```python
from build123d import *

# Parameters (mm, degrees)
BOSS_EXTRUDE1_DEPTH = 12.7
CUT_EXTRUDE1_DEPTH  = 10.795
SKETCH3_R           = 3.175
CUT_EXTRUDE2_DEPTH  = 23.622
SKETCH4_R           = 1.905
CUT_EXTRUDE3_DEPTH  = 7.62
SKETCH5_R           = 4.445
CUT_EXTRUDE4_DEPTH  = 1.27


with BuildPart() as part:
    # Sketch1 → Boss-Extrude1 (new body)
    with BuildSketch(Plane.XY):
        with BuildLine():
            Line((-15.875, 241.3), (-15.875, 41.885940063))
            ThreePointArc((-15.875, 41.885940063), (-17.859739298, 27.82498979), (-23.658870968, 14.862752926))
            ThreePointArc((-23.658870968, 14.862752926), (0, -27.94), (23.658870968, 14.862752926))
            ThreePointArc((23.658870968, 14.862752926), (17.859739298, 27.82498979), (15.875, 41.885940063))
            Line((15.875, 41.885940063), (15.875, 241.3))
            ThreePointArc((15.875, 241.3), (0, 257.175), (-15.875, 241.3))
        make_face()
    extrude(amount=BOSS_EXTRUDE1_DEPTH)

    # Sketch2 → Cut-Extrude1 (cut)
    with BuildSketch(Plane.XY.offset(12.7)):
        with BuildLine():
            Line((-11.43, 234.95), (11.43, 234.95))
            ThreePointArc((11.43, 234.95), (13.226051224, 234.206051224), (13.97, 232.41))
            Line((13.97, 232.41), (13.97, 41.885940063))
            ThreePointArc((13.97, 41.885940063), (16.029167022, 27.297704155), (22.045766129, 13.849383408))
            ThreePointArc((22.045766129, 13.849383408), (0, -26.035), (-22.045766129, 13.849383408))
            ThreePointArc((-22.045766129, 13.849383408), (-16.029167022, 27.297704155), (-13.97, 41.885940063))
            Line((-13.97, 41.885940063), (-13.97, 232.41))
            ThreePointArc((-13.97, 232.41), (-13.226051224, 234.206051224), (-11.43, 234.95))
        make_face()
    extrude(amount=-CUT_EXTRUDE1_DEPTH, mode=Mode.SUBTRACT)

    # Sketch3 → Cut-Extrude2 (cut)
    with BuildSketch(Plane.XY.offset(12.7)):
        with Locations((0, 241.3)):
            Circle(SKETCH3_R)
    extrude(amount=-CUT_EXTRUDE2_DEPTH, mode=Mode.SUBTRACT)

    # Sketch4 → Cut-Extrude3 (cut)
    with BuildSketch(Plane.XY.offset(12.7)):
        with Locations((-11.405580841, 241.3)):
            Circle(SKETCH4_R)
        with Locations((-9.877522754, 247.002790421)):
            Circle(SKETCH4_R)
        with Locations((-5.702790421, 251.177522754)):
            Circle(SKETCH4_R)
        with Locations((0, 252.705580841)):
            Circle(SKETCH4_R)
        with Locations((5.702790421, 251.177522754)):
            Circle(SKETCH4_R)
        with Locations((9.877522754, 247.002790421)):
            Circle(SKETCH4_R)
        with Locations((11.405580841, 241.3)):
            Circle(SKETCH4_R)
    extrude(amount=-CUT_EXTRUDE3_DEPTH, mode=Mode.SUBTRACT)

    # Sketch5 → Cut-Extrude4 (cut)
    with BuildSketch(Plane(origin=(0, 0, 0), x_dir=(-1, 0, 0), z_dir=(0, 0, -1))):
        with Locations((0, 241.3)):
            Circle(SKETCH5_R)
    extrude(amount=-CUT_EXTRUDE4_DEPTH, mode=Mode.SUBTRACT)


solid = part.part
```
Read the model definition and answer for the solid it produces. Units are mm, in the model's axes. A direction names the side the tool comes from. Give positions to 0.01 mm unless a question says otherwise; leave off trailing zeros. Order: outer loops, then holes, each group sorted by start corner. A loop starts at its lowest first (then second) coordinate and runs counter-clockwise, first axis right, second up. Notation, with made-up numbers: (77, 68) -> (126, 68) arc R6 ccw to (126, 79) -> close; hole circle Ø9 at (86.5, 65.5). An arc over 180 degrees is marked (long way). One line per item, written item: value. Start each with the question number.
(1) Straight lines are drawn through the part: L1, parallel to X at y = 241.3, z = 8 (3 decimals); L2, parallel to Y at x = 0, z = 2.75 (3 decimals); L3, parallel to X at y = 143, z = 6.5 (3 decimals). For each, find the intervals that lie inside material, in ascending order.
(2) Flat-ended cylindrical pins translate along their axes: P1, Ø1.1, axis at x = -10.5, y = 241.5, coming from the +Z side; P2, Ø4, axis at y = 124.5, z = 4.5, coming from the +X side (3 decimals); P3, Ø1.5, axis at y = 37, z = 8, coming from the +X side; P4, Ø2.5, axis at x = -1, y = 242.5, coming from the -Z side. Find the tip coordinate at first contact, or state that the pin passes through.
(3) The part is cut by section A-A (z = 9.25). State how many separate pieces and enclosed holes the cut face has, and give its area (3 significant figures).
(4) A tool of negligible diameter and unlimited length cuts with its end or side. For faces 1 (the flat face through (15.875, 140, 6)), 2 (the cylindrical face through (0.35, 257.17, 6.26)), 3 (the cylindrical face through (-16.087, 27.099, 7.378)), 4 (the flat face through (-3, 239, 1.27)), 5 (the flat face through (0, 85, 0)), from which of +Z, -Z, +X, -X, +Y, -Y can it reach the whole face along a straight path? Write none if from no direction.
(5) The part is cut by section B-B (y = 141). Determine the outline of the cut face in (x, z) (3 decimals), and give its area (3 significant figures).
(6) The part is cut by section C-C (x = -19). Determine the outline of the cut face in (y, z) (3 decimals).
(7) For a pull along Y with two mould halves and no side action, classify faces 6 (the cylindrical face through (-0.41, 244.45, 7.07)), 7 (the flat face through (0, 234.95, 7)), 8 (the flat face through (-15.875, 143, 6)), 9 (the cylindrical face through (-17.805, 28.017, 6.261)) as released by +Y, released by -Y, zero draft, split by the parting line, or undercut.
Taken from the geometry:
1. L1: -15.875 to -13.311, -9.501 to -3.175, 3.175 to 9.501, 13.311 to 15.875
1. L2: -27.94 to -26.035, 234.95 to 238.125, 244.475 to 257.175
1. L3: -15.875 to -13.97, 13.97 to 15.875
2. P1: z = 5.08
2. P2: x = 15.875
2. P3: x = 16.19
2. P4: through
3. separate pieces: 1
3. enclosed holes: 9
3. area: 1,550 mm^2
4. face 1: +Z, -Z, +X, +Y
4. face 2: +Z, -Z, +Y
4. face 3: +Z
4. face 4: -Z
4. face 5: -Z, +X, -X, +Y, -Y
5. outline: (-15.875, 0) -> (15.875, 0) -> (15.875, 12.7) -> (13.97, 12.7) -> (13.97, 1.905) -> (-13.97, 1.905) -> (-13.97, 12.7) -> (-15.875, 12.7) -> close
5. area: 102 mm^2
6. outline: (-20.485, 0) -> (24.344, 0) -> (24.344, 12.7) -> (19.416, 12.7) -> (19.416, 1.905) -> (-17.799, 1.905) -> (-17.799, 12.7) -> (-20.485, 12.7) -> close
7. face 6: undercut
7. face 7: undercut
7. face 8: zero draft
7. face 9: released by +Y
